Geometry check sheet. Reference: the model listing, model coordinates, mm. Face numbers are marked on the shaded views. A direction names the side the tool comes from. Coordinates: 2 decimals unless noted, no trailing zeros. Write each loop counter-clockwise with the first axis right and the second up, starting at its lowest first coordinate (ties: lowest second). Pieces come first, ordered by that corner, then holes.
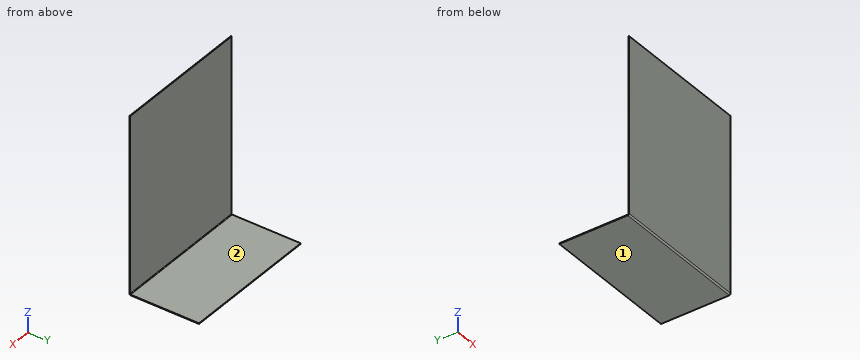
from build123d import *

# Parameters (mm, degrees)
SKETCH1_W          = 203.2
SKETCH1_H          = 254
BASE_FLANGE1_DEPTH = 1
EDGE_FLANGE1_DEPTH = 203.2


# Sheet-metal steps are written as plain solids
with BuildPart() as part:
    # Sketch1 → Base-Flange1 (new body)
    with BuildSketch(Plane(origin=(0, 0, 0), x_dir=(1, 0, 0), z_dir=(0, 1, 0))):
        Rectangle(SKETCH1_W, SKETCH1_H)
    extrude(amount=-BASE_FLANGE1_DEPTH)

    # Edge-Flange1 section (across the edge) → Edge-Flange1 (add)
    with BuildSketch(Plane(origin=(101.6, 0, -130), x_dir=(0, 0, 1), z_dir=(-1, 0, 0))):
        with BuildLine():
            Line((0, 1), (0, 100.6))
            Line((0, 100.6), (1, 100.6))
            Line((1, 100.6), (1, 1))
            ThreePointArc((1, 1), (1.292893219, 0.292893219), (2, 0))
            Line((2, 0), (3, 0))
            Line((3, 0), (3, -1))
            Line((3, -1), (2, -1))
            ThreePointArc((2, -1), (0.585786438, -0.414213562), (0, 1))
        make_face()
    extrude(amount=EDGE_FLANGE1_DEPTH)


solid = part.part
1. Access from +Z, -Z, +X, -X, +Y, -Y to the whole of each face (thin tool, end or side, straight path). Record for the marked faces 1 and 2.
Computed values:
face 1: -Z, +X, -X, +Y, -Y
face 2: +Z, +X, -X, +Y
2. Sectioned sample at A-A, the plane x = -37. Record the boundary of the cut face in (y, z), and give its area (3 significant figures).
Computed values:
outline: (-1, -128) arc R2 ccw to (1, -130) - (100.6, -130) - (100.6, -129) - (1, -129) arc R1 cw to (0, -128) - (0, 127) - (-1, 127) - close
area: 357 mm2
3. Gauge pin test, flat ends, axial feed: pin 1 Ø1.5 at (x, y) = (55.5, 40) entering from +Z; pin 2 Ø10 at (x, z) = (-77.5, 67) entering from +Y. Record the tip position at first contact, or that the pin passes through.
Computed values:
pin 1: stops at z = -129
pin 2: stops at y = 0
4. Sectioned sample at C-C, the plane z = 39.5. Record the boundary of the cut face in (x, y), and give its area (3 significant figures).
Computed values:
outline: (-101.6, -1) - (101.6, -1) - (101.6, 0) - (-101.6, 0) - close
area: 203 mm2
5. Thickness scan on line 1 along Y through (x, z) = (40.5, 9.5); line 2 along Z through (x, y) = (-64, 65). Record the ranges inside material, lowest first.
Computed values:
line 1: y = -1 to 0
line 2: z = -130 to -129
6. Sectioned sample at B-B, the plane y = 42. Record the boundary of the cut face in (x, z).
Computed values:
outline: (-101.6, -130) - (101.6, -130) - (101.6, -129) - (-101.6, -129) - close
